Read the model definition and answer for the solid it produces. Units are mm, in the model's axes. Face numbers are marked on the shaded views. A direction names the side the tool comes from. Give positions to 0.01 mm unless a question says otherwise; leave off trailing zeros. Loops run counter-clockwise (first coordinate to the right, second up) from the corner with the lowest first, then second, coordinate; pieces in that order, holes last.
(1) Find section D-D, the plane z = 1. Write down the section's boundary in (x, y), then the cut area to 3 significant figures.
(2) Find section C-C, the plane x = 0. Write down the section's boundary in (y, z), then the cut area to 3 significant figures.
(3) Find section B-B, the plane z = 2.75. Write down the section's boundary in (x, y).
(4) Determine the mould class of the marked faces 1, 2, 3 and 4 for opening direction Y: pulls with the +Y half, pulls with the -Y half, needs draft (parallel to the pull), parting line crosses it, or undercut.
(5) Find section A-A, the plane y = -11.5. Write down the section's boundary in (x, z).
(6) Straight lines are drawn through the part: probe 1 along X at (y, z) = (-8.25, 4.25); probe 2 along Z at (x, y) = (12.75, -11.5); probe 3 along Y at (x, z) = (0, 1.65). For each, find the intervals that lie inside material, in ascending order.
(7) Each of these flat-tipped pins is pushed along its axis until it touches: P1, Ø11, axis at x = 4.5, y = 0, coming from the +Z side; P2, Ø4.5, axis at x = 14.5, z = 3, coming from the +Y side; P3, Ø2.5, axis at x = 0, y = 1, coming from the +Z side; P4, Ø3, axis at x = -14.5, z = 4, coming from the +Y side. Where does it stop, or does it pass through?
(8) Which of the six approach directions +Z, -Z, +X, -X, +Y, -Y give full straight-line access (tool end or side, diameter ignored) to the marked faces 5, 6 and 7?
```python
from build123d import *

# Parameters (mm, degrees)
PAD_DEPTH       = 2
PAD001_DEPTH    = 35
SKETCH002_R     = 1.6
POCKET_DEPTH    = 35.001
SKETCH003_W     = 20
SKETCH003_H     = 10
POCKET001_DEPTH = 22.001
FILLET_R        = 3
SKETCH004_R     = 1.65
POCKET002_DEPTH = 5


with BuildPart() as part:
    # Sketch → Pad (new body)
    with BuildSketch(Plane.XY):
        Polygon((-17.5, -15), (17.5, -15), (17.5, -7), (11, 7), (-11, 7), (-17.5, -7), align=None)
    extrude(amount=PAD_DEPTH)

    # Sketch001 (on Face6 of Pad) → Pad001 (join)
    with BuildSketch(Plane(origin=(-17.5, 0, 0), x_dir=(0, -1, 0), z_dir=(-1, 0, 0))):
        with BuildLine():
            Line((15, 2), (15, 6))
            ThreePointArc((15, 6), (11.5, 9.5), (8, 6))
            Line((8, 2), (8, 6))
            Line((8, 2), (15, 2))
        make_face()
    extrude(amount=-PAD001_DEPTH)

    # Sketch002 (on Face8 of Pad001) → Pocket (cut, through all)
    with BuildSketch(Plane(origin=(-17.5, 0, 0), x_dir=(0, -1, 0), z_dir=(-1, 0, 0))):
        with Locations((11.5, 6)):
            Circle(SKETCH002_R)
    extrude(amount=-POCKET_DEPTH, mode=Mode.SUBTRACT)

    # Sketch003 (on Face1 of Pocket) → Pocket001 (cut, through all)
    with BuildSketch(Plane.XZ.offset(15)):
        with Locations((0, 7)):
            Rectangle(SKETCH003_W, SKETCH003_H)
    extrude(amount=-POCKET001_DEPTH, mode=Mode.SUBTRACT)

    # Fillet
    fillet_edges = [part.edges().sort_by_distance(p)[0] for p in [
        (-11, 7, 1),
        (-17.5, -7, 1),
        (11, 7, 1),
        (17.5, -7, 1),
    ]]
    fillet(fillet_edges, radius=FILLET_R)

    # Sketch004 (on Face2 of Fillet) → Pocket002 (cut)
    with BuildSketch(Plane(origin=(0, 0, 0), x_dir=(1, 0, 0), z_dir=(0, 0, -1))):
        with Locations((0, -1)):
            Circle(SKETCH004_R)
    extrude(amount=-POCKET002_DEPTH, mode=Mode.SUBTRACT)


solid = part.part
```
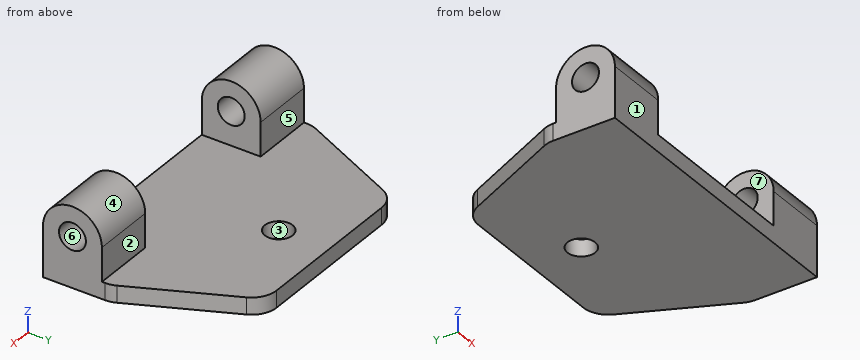
Entries:
1. outline: (-17.5, -15) - (17.5, -15) - (17.5, -7.66) arc R3 ccw to (17.22, -6.4) - (11.81, 5.26) arc R3 ccw to (9.09, 7) - (-9.09, 7) arc R3 ccw to (-11.81, 5.26) - (-17.22, -6.4) arc R3 ccw to (-17.5, -7.66) - close; hole circle Ø3.3 at (0, 1)
1. area: 669 mm2
2. outline: (-15, 0) - (-0.65, 0) - (-0.65, 2) - (-15, 2) - close; (2.65, 0) - (7, 0) - (7, 2) - (2.65, 2) - close
2. area: 37.4 mm2
3. outline: (-17.5, -15) - (-10, -15) - (-10, -8) - (-17.5, -8) - close; (10, -15) - (17.5, -15) - (17.5, -8) - (10, -8) - close
4. face 1: pulls with the -Y half
4. face 2: pulls with the +Y half
4. face 3: undercut
4. face 4: parting line crosses it
5. outline: (-17.5, 0) - (17.5, 0) - (17.5, 4.4) - (10, 4.4) - (10, 2) - (-10, 2) - (-10, 4.4) - (-17.5, 4.4) - close; (-17.5, 7.6) - (-10, 7.6) - (-10, 9.5) - (-17.5, 9.5) - close; (10, 7.6) - (17.5, 7.6) - (17.5, 9.5) - (10, 9.5) - close
6. probe 1: x = -17.5 to -10, 10 to 17.5
6. probe 2: z = 0 to 4.4, 7.6 to 9.5
6. probe 3: y = -15 to -0.65, 2.65 to 7
7. P1: stops at z = 2
7. P2: stops at y = 3.8
7. P3: passes through
7. P4: stops at y = -8
8. face 5: +Z, +X, -X, +Y
8. face 6: +X, -X
8. face 7: +Z, +Y, -Y
